Autodesk Inventor part; units mm, degrees
ref_plane "YZ Plane" through (0, 0, 0) normal (1, 0, 0) x (0, 1, 0)
ref_plane "XZ Plane" through (0, 0, 0) normal (0, 1, 0) x (-1, 0, 0)
ref_plane "XY Plane" through (0, 0, 0) normal (0, 0, 1) x (1, 0, 0)
sketch "Sketch1" plane through (0, 0, 0) normal (0, 1, 0) x (-1, 0, 0)
  line L0 (-36.0847, -75.9608) -> (-36.0847, -87.9608)
  line L1 (-36.0847, -87.9608) -> (42.9536, -87.9608)
  line L2 (42.9536, -87.9608) -> (42.9536, -75.9608)
  line L3 (42.9536, -75.9608) -> (-36.0847, -75.9608)
  line L4 (-36.0847, -75.9608) -> (-36.0847, -87.9608)
  circle A0 centre (-18.6075, -81.9608) radius 1.4
  circle A1 centre (-18.6075, -81.9608) radius 1.4
  circle A2 centre (6.6962, -81.9608) radius 1.4
  circle A3 centre (6.6962, -81.9608) radius 1.4
  circle A4 centre (37.2679, -81.9608) radius 1.4
  circle A5 centre (37.2679, -81.9608) radius 1.4
  line L5 (-36.0847, 90.7296) -> (-36.0847, 102.7296)
  line L6 (-36.0847, 102.7296) -> (42.9536, 102.7296)
  line L7 (42.9536, 102.7296) -> (42.9536, 90.7296)
  line L8 (42.9536, 90.7296) -> (-36.0847, 90.7296)
  line L9 (-36.0847, 90.7296) -> (-36.0847, 102.7296)
  circle A6 centre (-18.6075, 96.7296) radius 1.4
  circle A7 centre (-18.6075, 96.7296) radius 1.4
  circle A8 centre (6.6962, 96.7296) radius 1.4
  circle A9 centre (6.6962, 96.7296) radius 1.4
  circle A10 centre (37.2679, 96.7296) radius 1.4
  circle A11 centre (37.2679, 96.7296) radius 1.4
  point P0 (0, 0)
  point P1 (-48.8522, 7.3844)
extrude "Extrusion1" add sketch "Sketch1" along normal blind 3
sketch "Sketch2" plane through (0, 3, 0) normal (0, 1, 0) x (1, 0, 0)
  line L0 (36.0847, -90.7296) -> (-42.9536, -90.7296)
  line L1 (-42.9536, -90.7296) -> (-42.9536, -102.7296)
  line L2 (36.0847, -90.7296) -> (-42.9536, -90.7296)
  line L3 (-42.9536, -90.7296) -> (-42.9536, -93.7296)
  line L4 (-42.9536, -93.7296) -> (36.0847, -93.7296)
  line L5 (36.0847, -93.7296) -> (36.0847, -90.7296)
  line L6 (-42.9536, 76.0091) -> (36.0847, 76.0091)
  line L7 (36.0847, 76.0091) -> (36.0847, 79.0091)
  line L8 (36.0847, 79.0091) -> (-42.9536, 79.0091)
  line L9 (-42.9536, 79.0091) -> (-42.9536, 76.0091)
  point P0 (0, 0)
  dimension "d2" = 3
  dimension "d3" = 3
extrude "Extrusion2" add sketch "Sketch2" along normal blind 25
sketch "Sketch3" plane through (-42.9536, 3, -76.0091) normal (0, 0, 1) x (1, 0, 0)
  line L0 (0, 0) -> (0, 25)
  line L1 (79.0383, 0) -> (79.0383, 25)
  line L2 (0, 25) -> (79.0383, 25)
  line L3 (79.0383, 25) -> (79.0383, 20)
  line L4 (79.0383, 20) -> (0, 20)
  line L5 (0, 20) -> (0, 25)
  point P0 (42.9536, -3)
  point P1 (0, 20)
  dimension "d6" = 5
extrude "Extrusion3" add sketch "Sketch3" along normal blind 168
sketch "Sketch4" plane through (-42.9536, 3, 93.7296) normal (0, 0, 1) x (1, 0, 0)
  line L0 (79.0383, 0) -> (0, 0)
  line L1 (22.5307, 0) -> (52.1586, 0)
  line L2 (52.1586, 0) -> (52.1586, 14.1048)
  line L3 (52.1586, 14.1048) -> (22.5307, 14.1048)
  line L4 (22.5307, 14.1048) -> (22.5307, 0)
  point P0 (42.9536, -3)
extrude "Extrusion4" cut sketch "Sketch4" against normal blind 20
sketch "Sketch5" plane through (36.0847, 0, 102.7296) normal (1, 0, 0) x (0, 0, -1)
  line L0 (0, 3) -> (9, 3)
  line L1 (0, 3) -> (9, 14.3829)
  line L2 (9, 3) -> (9, 28)
  line L3 (0, 0) -> (0, 3)
  line L4 (0, 3) -> (9, 3)
  line L5 (9, 14.3829) -> (9, 3)
  point P0 (102.7296, 0)
extrude "Extrusion5" add sketch "Sketch5" against normal blind 5
sketch "Sketch7" plane through (36.0847, 0, 102.7296) normal (1, 0, 0) x (0, 0, -1)
  line L0 (190.7387, 3) -> (181.7387, 14.3829)
  line L1 (181.7387, 14.3829) -> (190.7387, 3)
  line L2 (181.7387, 3) -> (190.7387, 3)
  line L3 (190.7387, 3) -> (181.7387, 3)
  line L4 (181.7387, 3) -> (181.7387, 14.3829)
  point P0 (102.7296, 0)
extrude "Extrusion7" add sketch "Sketch7" against normal blind 5
sketch "Sketch10" plane through (36.0847, 3, -76.0091) normal (0, 0, 1) x (1, 0, 0)
  line L0 (0, -3) -> (0, 0)
  line L1 (0, 20) -> (-79.0383, 20)
  line L2 (0, -3) -> (-5, -3)
  line L3 (-5, -3) -> (-5, 20)
  line L4 (-5, 20) -> (0, 20)
  line L5 (0, 20) -> (0, -3)
  point P0 (-36.0847, -3)
  point P1 (-74.0383, 20)
  dimension "d22" = 5
extrude "Extrusion10" add sketch "Sketch10" along normal blind 168
sketch "Sketch11" plane through (0, 28, 0) normal (0, 1, 0) x (1, 0, 0)
  line L0 (-42.9536, 79.0091) -> (-42.9536, -93.7296)
  line L1 (-42.9536, -7.3603) -> (36.0847, -7.3603)
  line L2 (36.0847, -93.7296) -> (36.0847, 79.0091)
  point P0 (0, 0)
sketch "Sketch12" plane through (-42.9536, 0, -87.9608) normal (-1, 0, 0) x (0, 0, 1)
  line L0 (0, 0) -> (190.6905, 0)
  line L1 (0, 0) -> (0, 3)
  line L2 (0, 0) -> (0, 3)
  point P0 (87.9608, 0)
sketch "Sketch13" plane through (-42.9536, 0, 90.7296) normal (-1, 0, 0) x (0, 0, 1)
  line L0 (-178.6905, 0) -> (-178.6905, 3)
  line L1 (-178.6905, 0) -> (-178.6905, 3)
  line L2 (-169.7387, 3) -> (-169.7387, 28)
  line L3 (-178.6905, 3) -> (-169.7387, 3)
  line L4 (-169.7387, 28) -> (3, 28)
  line L5 (-169.7387, 3) -> (-169.7387, 28)
  line L6 (-169.7387, 28) -> (3, 28)
  line L7 (3, 28) -> (3, 3)
  line L8 (12, 0) -> (12, 3)
  line L9 (3, 3) -> (12, 3)
  line L10 (12, 3) -> (12, 0)
  line L11 (0, 23) -> (0, 0)
  line L12 (12, 0) -> (0, 0)
  line L13 (0, 0) -> (0, 23)
  line L14 (-166.7387, 3) -> (-166.7387, 23)
  line L15 (0, 23) -> (-166.7387, 23)
  line L16 (-166.7387, 23) -> (-166.7387, 0)
  line L17 (-166.7387, 0) -> (-178.6905, 0)
  point P0 (-90.7296, 0)
extrude "Extrusion11" add sketch "Sketch13" along normal blind 3.5
sketch "Sketch14" plane through (-46.4536, 0, 90.7296) normal (-1, 0, 0) x (0, 0, 1)
  line L0 (-169.7387, 14.3829) -> (-178.7387, 3)
  line L1 (12, 3) -> (3, 14.3829)
  line L2 (-169.7387, 3) -> (-178.6905, 3)
  line L3 (-178.7387, 3) -> (-169.7387, 3)
  line L4 (-169.7387, 3) -> (-169.7387, 14.3829)
  line L5 (-169.7387, 14.3829) -> (-178.7387, 3)
  line L6 (3, 14.3829) -> (3, 3)
  line L7 (3, 3) -> (12, 3)
  line L8 (3, 14.3829) -> (12, 3)
  point P0 (-90.7296, 0)
extrude "Extrusion12" add sketch "Sketch14" against normal blind 5
sketch "Sketch15" plane through (31.0847, 0, 90.7296) normal (0, 0, -1) x (-1, 0, 0)
  line L0 (77.5383, 23) -> (77.5383, 0)
  line L1 (0, 0) -> (77.5383, 0)
  line L2 (77.5383, 23) -> (72.5383, 23)
  line L3 (72.5383, 23) -> (72.5383, 0)
  line L4 (72.5383, 0) -> (77.5383, 0)
  line L5 (77.5383, 0) -> (77.5383, 23)
  point P0 (31.0847, 0)
  dimension "d29" = 5
extrude "Extrusion13" add sketch "Sketch15" along normal blind 168
sketch "Sketch16" plane through (0, 28, 0) normal (0, 1, 0) x (1, 0, 0)
  line L0 (31.0847, 75.9608) -> (31.0847, -90.7296)
  circle A0 centre (31.0847, 72.801) radius 1.65
  circle A1 centre (-37.2679, 72.801) radius 1.65
  circle A2 centre (-6.278, 72.801) radius 1.65
  line L1 (-42.9536, -7.3603) -> (36.0847, -7.3603)
  circle A3 centre (31.0847, -87.5216) radius 1.65
  circle A4 centre (-37.2679, -87.5216) radius 1.65
  circle A5 centre (-6.278, -87.5216) radius 1.65
  point P0 (0, 0)
  point P1 (31.0847, -90.6814)
  dimension "d32" = 3.3
  dimension "d33" = 3.3
extrude "Extrusion14" cut sketch "Sketch16" against normal blind 168
sketch "Sketch17" plane through (0, 28, 0) normal (0, 1, 0) x (1, 0, 0)
  line L0 (36.0847, 79.0091) -> (-46.4536, 79.0091)
  line L1 (31.0847, -93.7296) -> (36.0847, -93.7296)
  line L2 (-46.4536, 79.0091) -> (36.0847, 79.0091)
  line L3 (36.0847, 79.0091) -> (36.0847, -93.7296)
  line L4 (36.0847, -93.7296) -> (-46.4536, -93.7296)
  line L5 (-46.4536, -93.7296) -> (-46.4536, 79.0091)
  arc A0 (31.0847, -89.1716) -> (31.0847, -85.8716) centre (31.0847, -87.5216) ccw
  circle A1 centre (31.0847, -87.5216) radius 1.65
  circle A2 centre (-6.278, -87.5216) radius 1.65
  circle A3 centre (-6.278, -87.5216) radius 1.65
  circle A4 centre (-37.2679, -87.5216) radius 1.65
  circle A5 centre (-37.2679, -87.5216) radius 1.65
  circle A6 centre (-37.2679, 72.801) radius 1.65
  circle A7 centre (-37.2679, 72.801) radius 1.65
  circle A8 centre (-6.278, 72.801) radius 1.65
  circle A9 centre (-6.278, 72.801) radius 1.65
  arc A10 (31.0847, 71.151) -> (31.0847, 74.451) centre (31.0847, 72.801) ccw
  circle A11 centre (31.0847, 72.801) radius 1.65
  point P0 (0, 0)
  point P1 (31.0847, -85.8716)
extrude "Extrusion15" cut sketch "Sketch17" against normal blind 10
sketch "Sketch18" plane through (-41.4536, 0, 90.7296) normal (1, 0, 0) x (0, 0, -1)
  line L0 (166.7387, 18) -> (0, 18)
  line L1 (166.7387, 18) -> (166.7387, 3)
  line L2 (0, 18) -> (166.7387, 18)
  line L3 (166.7387, 18) -> (166.7387, 13)
  line L4 (166.7387, 13) -> (0, 13)
  line L5 (0, 13) -> (0, 18)
  point P0 (90.7296, 0)
  dimension "d38" = 5
extrude "Extrusion16" add sketch "Sketch18" along normal blind 75
sketch "Sketch19" plane through (0, 18, 0) normal (0, 1, 0) x (1, 0, 0)
  line L0 (33.4512, -7.3603) -> (-16.5488, -7.3603)
  line L1 (-16.5488, -7.3603) -> (-16.5488, 69.1397)
  line L2 (-16.5488, 69.1397) -> (33.4512, 69.1397)
  line L3 (33.4512, 69.1397) -> (33.4512, -7.3603)
  line L4 (33.4512, -7.3603) -> (-16.5488, -7.3603)
  line L5 (-16.5488, -7.3603) -> (-16.5488, -83.8603)
  line L6 (-16.5488, -83.8603) -> (33.4512, -83.8603)
  line L7 (33.4512, -83.8603) -> (33.4512, -7.3603)
  line L8 (36.0847, 79.0091) -> (36.0847, -93.7296)
  line L9 (36.0847, -7.3603) -> (-18.6839, -7.3603)
  line L10 (-18.6839, -7.3603) -> (-18.6839, -86.5599)
  line L11 (-18.6839, -86.5599) -> (36.0847, -86.5599)
  line L12 (36.0847, -86.5599) -> (36.0847, -7.3603)
  line L13 (-18.6839, 71.8393) -> (36.0847, 71.8393)
  line L14 (-18.6839, -7.3603) -> (-18.6839, 71.8393)
  circle A0 centre (-11.398, -90.2259) radius 1.65
  circle A1 centre (25.0886, -90.2259) radius 1.65
  line L15 (36.0847, -86.5599) -> (36.0847, -93.7296)
  line L16 (36.0847, -93.7296) -> (-18.6839, -93.7296)
  line L17 (-20.4229, -90.7296) -> (9.205, -90.7296)
  line L18 (-18.6839, -93.7296) -> (-18.6839, -86.5599)
  line L19 (-18.6839, 71.8393) -> (36.0847, 71.8393)
  circle A2 centre (-11.398, 75.5053) radius 1.65
  circle A3 centre (25.0886, 75.5053) radius 1.65
  line L20 (36.0847, 71.8393) -> (36.0847, 79.0091)
  line L21 (36.0847, 79.0091) -> (-18.6839, 79.0091)
  line L22 (-20.4229, 76.0091) -> (9.205, 76.0091)
  line L23 (-18.6839, 79.0091) -> (-18.6839, 71.8393)
  point P0 (0, 0)
  dimension "d41" = 50
  dimension "d42" = 76.5
  dimension "d43" = 76.5
  dimension "d44" = 3.3
  dimension "d45" = 3.3
extrude "Extrusion17" cut sketch "Sketch19" against normal blind 75 contours A2 L22 | L22 A2 | A0 L17 | L17 A0 | A1 | A3
sketch "Sketch20" plane through (0, 18, 0) normal (0, 1, 0) x (1, 0, 0)
  circle A0 centre (-11.398, 75.5053) radius 1.65
  line L0 (-11.398, 75.5053) -> (-37.0391, 75.5053)
  line L1 (-12.9693, 76.0091) -> (-41.4536, 76.0091)
  circle A1 centre (-37.0391, 75.5053) radius 1.65
  line L2 (-42.9536, -7.3603) -> (36.0847, -7.3603)
  circle A2 centre (-37.0391, -90.2259) radius 1.65
  line L3 (-46.4536, -93.7296) -> (-46.4536, 79.0091)
  line L4 (-46.4536, -7.3603) -> (-19.4536, -7.3603)
  line L5 (-19.4536, -7.3603) -> (-40.4536, -7.3603)
  line L6 (-40.4536, -7.3603) -> (-40.4536, 47.6397)
  line L7 (-40.4536, 47.6397) -> (-19.4536, 47.6397)
  line L8 (-19.4536, 47.6397) -> (-19.4536, -7.3603)
  line L9 (-19.4536, -7.3603) -> (-40.4536, -7.3603)
  line L10 (-40.4536, -7.3603) -> (-40.4536, -62.3603)
  line L11 (-40.4536, -62.3603) -> (-19.4536, -62.3603)
  line L12 (-19.4536, -62.3603) -> (-19.4536, -7.3603)
  circle A3 centre (-29.9536, 52.2555) radius 1.65
  line L13 (-29.9536, -62.3603) -> (-29.9536, -66.9763)
  circle A4 centre (-29.9536, -66.9763) radius 1.65
  line L14 (-19.4536, -72.5437) -> (-40.4536, -72.5437)
  line L15 (-40.4536, -72.5437) -> (-40.4536, -83.7487)
  line L16 (-40.4536, -83.7487) -> (-19.4536, -83.7487)
  line L17 (-19.4536, -83.7487) -> (-19.4536, -72.5437)
  line L18 (-19.4536, 57.8231) -> (-40.4536, 57.8231)
  line L19 (-40.4536, 57.8231) -> (-40.4536, 69.0282)
  line L20 (-40.4536, 69.0282) -> (-19.4536, 69.0282)
  line L21 (-19.4536, 69.0282) -> (-19.4536, 57.8231)
  point P0 (0, 0)
  point P1 (-41.4536, -90.7296)
  dimension "d48" = 3.3
  dimension "d49" = 27
  dimension "d50" = 21
  dimension "d51" = 55
  dimension "d52" = 55
  dimension "d53" = 3.3
  dimension "d54" = 4.616
  dimension "d55" = 3.3
extrude "Extrusion18" cut sketch "Sketch20" against normal blind 75 contours A4 | A3 | L17 L16 L15 L14 | L18 L19 L20 L21
sketch "Sketch21" plane through (0, 18, 0) normal (0, 1, 0) x (1, 0, 0)
  line L0 (-42.9536, -7.3603) -> (36.0847, -7.3603)
  line L1 (-29.9536, -7.3603) -> (-17.4536, -7.3603)
  line L2 (-17.4536, -7.3603) -> (-17.4536, -62.3603)
  line L3 (-17.4536, -62.3603) -> (-29.9536, -62.3603)
  line L4 (-29.9536, -62.3603) -> (-29.9536, -7.3603)
  line L5 (-29.9536, -7.3603) -> (-42.4536, -7.3603)
  line L6 (-42.4536, -7.3603) -> (-42.4536, -62.3603)
  line L7 (-42.4536, -62.3603) -> (-29.9536, -62.3603)
  line L8 (-17.4536, -7.3603) -> (-17.4536, 47.6397)
  line L9 (-17.4536, 47.6397) -> (-29.9536, 47.6397)
  line L10 (-29.9536, 47.6397) -> (-29.9536, -7.3603)
  line L11 (-42.4536, -7.3603) -> (-42.4536, 47.6397)
  line L12 (-42.4536, 47.6397) -> (-29.9536, 47.6397)
  line L13 (-17.4536, 47.6397) -> (-42.4536, 47.6397)
  line L14 (-42.4536, 47.6397) -> (-42.4536, 56.0699)
  line L15 (-42.4536, 56.0699) -> (-17.4536, 56.0699)
  line L16 (-17.4536, 56.0699) -> (-17.4536, 47.6397)
  line L17 (-17.4536, -62.3603) -> (-29.9536, -62.3603)
  line L18 (-42.4536, -62.3603) -> (-29.9536, -62.3603)
  line L19 (-17.4536, -62.3603) -> (-42.4536, -62.3603)
  line L20 (-42.4536, -62.3603) -> (-42.4536, -70.7904)
  line L21 (-42.4536, -70.7904) -> (-17.4536, -70.7904)
  line L22 (-17.4536, -70.7904) -> (-17.4536, -62.3603)
  point P0 (0, 0)
  dimension "d58" = 12.5
  dimension "d59" = 55
properties part number "atap"
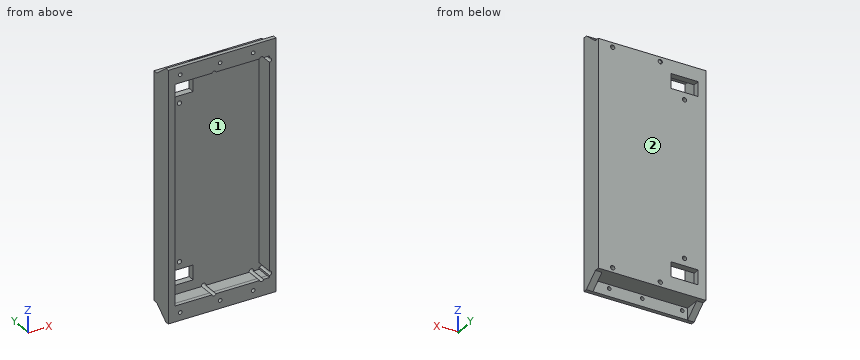
For this review, take the finished solid that the model builds, in its own axes (mm). Face numbers are marked on the shaded views. Give positions to 0.01 mm unless a question says otherwise; leave off trailing zeros. Write each loop counter-clockwise with the first axis right and the second up, starting at its lowest first coordinate (ties: lowest second). Pieces come first, ordered by that corner, then holes. Notation, with made-up numbers: M -18,18.25 L 8,18.25 A23 ccw 8,50.25 Z; hole C 28.5,85.25 d1. An arc over 180 degrees is marked long. Answer as a JSON object with one key per item and string values. Group by question number.
Item 1: Consider section A-A on x = -34. Write out the cut boundary in (y, z).
Item 2: Draft analysis for pull direction X (two halves, no side actions). For the marked faces 1 and 2, state which applies: +X half, -X half, draft (parallel to the pull), parting line (faces both ways), or undercut.
Item 3: For probe 1 along Z at (x, y) = (-37.5, 16.25); probe 2 along Z at (x, y) = (-38.5, 7.5); probe 3 along X at (y, z) = (5.25, 13), list the stretches that pass through material, from the lowest coordinate up. Write a range as [from, to].
Item 4: Consider section C-C on x = -2.5. Write out the cut boundary in (y, z).
Item 5: Consider section B-B on z = 29. Write out the cut boundary in (x, y).
Item 6: For pin 1 Ø6 at (x, y) = (-31, 12.5) entering from +Z; pin 2 Ø2.5 at (x, z) = (25.09, 90.23) entering from -Y; pin 3 Ø1 at (x, y) = (12.5, 13.5) entering from -Z; pin 4 Ø8 at (x, y) = (-6.5, 10) entering from +Z, all flat-tipped, find the tip position at first contact; note any pin that passes through.
Check result:
{
 "1": {"outline": "M 0,-87.96 L 3,-87.96 L 3,-79.01 L 18,-79.01 L 18,-69.03 L 13,-69.03 L 13,-76.01 L 3,-76.01 L 3,-75.96 L 0,-75.96 Z; M 0,90.73 L 13,90.73 L 13,83.75 L 18,83.75 L 18,93.73 L 3,93.73 L 3,102.73 L 0,102.73 Z; M 13,-57.82 L 18,-57.82 L 18,72.54 L 13,72.54 Z"},
 "2": {"face 1": "undercut", "face 2": "draft"},
 "3": {"probe 1": "z = [-79.01, -69.03], [-57.82, 72.54], [83.75, 93.73]", "probe 2": "z = [-79.01, -76.01], [90.73, 93.73]", "probe 3": "x = [-46.45, -41.45], [31.08, 36.08]"},
 "4": {"outline": "M 0,-87.96 L 3,-87.96 L 3,-79.01 L 18,-79.01 L 18,93.73 L 17.1,93.73 L 17.1,90.73 L 13,90.73 L 13,-76.01 L 3,-76.01 L 3,-75.96 L 0,-75.96 Z; M 0,90.73 L 3,90.73 L 3,102.73 L 0,102.73 Z"},
 "5": {"outline": "M -46.45,0 L -41.45,0 L -41.45,13 L 31.08,13 L 31.08,0 L 36.08,0 L 36.08,18 L -46.45,18 Z"},
 "6": {"pin 1": "stops at z = 93.73", "pin 2": "passes through", "pin 3": "stops at z = -79.01", "pin 4": "stops at z = 90.73"}
}
